from build123d import *

# Parameters (mm, degrees)
BOSS_EXTRUDE1_DEPTH = 6
SKETCH2_R           = 2
CUT_EXTRUDE1_DEPTH  = 121.370262108
SKETCH3_R           = 2
CUT_EXTRUDE2_DEPTH  = 121.370262108
CUT_EXTRUDE3_DEPTH  = 4
SKETCH6_W           = 48
SKETCH6_H           = 40
CUT_EXTRUDE4_DEPTH  = 109.231233939
FILLET1_R           = 5
CHAMFER1_SIZE       = 1


with BuildPart() as part:
    # Sketch1 → Boss-Extrude1 (new, symmetric)
    with BuildSketch(Plane(origin=(0, 0, 0), x_dir=(1, 0, 0), z_dir=(0, 1, 0))):
        Polygon((20, 103), (31, 103), (31, 0), (-31, 0), (-31, 103), (-20, 103), (-20, 10), (20, 10), align=None)
    extrude(amount=BOSS_EXTRUDE1_DEPTH, both=True)

    # Sketch2 → Cut-Extrude1 (cut, through all)
    with BuildSketch(Plane(origin=(31, 0, 0), x_dir=(0, 0, -1), z_dir=(1, 0, 0))):
        with Locations((97, 0)):
            Circle(SKETCH2_R)
        with BuildLine():
            Line((97, 6), (104, 6))
            Line((104, 6), (104, -6))
            Line((104, -6), (97, -6))
            ThreePointArc((97, -6), (103, 0), (97, 6))
        make_face()
    extrude(amount=-CUT_EXTRUDE1_DEPTH, mode=Mode.SUBTRACT)

    # Sketch3 → Cut-Extrude2 (cut, through all)
    with BuildSketch(Plane(origin=(31, 0, 0), x_dir=(0, 0, -1), z_dir=(1, 0, 0))):
        with Locations((18, 0)):
            Circle(SKETCH3_R)
    extrude(amount=-CUT_EXTRUDE2_DEPTH, mode=Mode.SUBTRACT)

    # Sketch4 → Cut-Extrude3 (cut)
    with BuildSketch(Plane(origin=(31, 0, 0), x_dir=(0, 0, -1), z_dir=(1, 0, 0))):
        Polygon((22.041451884, 0), (20.020725942, 3.5), (15.979274058, 3.5), (13.958548116, 0), (15.979274058, -3.5), (20.020725942, -3.5), align=None)
    cut_extrude3 = extrude(amount=-CUT_EXTRUDE3_DEPTH, mode=Mode.SUBTRACT)

    # Mirror1: Cut-Extrude3 across plane
    add(cut_extrude3.mirror(Plane(origin=(0, 0, 0), x_dir=(0, 0, 1), z_dir=(1, 0, 0))), mode=Mode.SUBTRACT)

    # Sketch6 → Cut-Extrude4 (cut, through all)
    with BuildSketch(Plane(origin=(0, 6, 0), x_dir=(1, 0, 0), z_dir=(0, 1, 0))):
        with Locations((0, 30)):
            Rectangle(SKETCH6_W, SKETCH6_H)
    extrude(amount=-CUT_EXTRUDE4_DEPTH, mode=Mode.SUBTRACT)

    # Fillet1
    fillet1_edges = [part.edges().sort_by_distance(p)[0] for p in [
        (31, 0, 0),
        (-31, 0, 0),
    ]]
    fillet(fillet1_edges, radius=FILLET1_R)

    # Chamfer1
    chamfer1_edges = [part.edges().sort_by_distance(p)[0] for p in [
        (-20, -6, -73.5),
        (-20, 6, -73.5),
        (0, -6, 0),
        (0, 6, 0),
        (31, -6, -51),
        (29.535533906, -6, -1.464466094),
        (-29.535533906, -6, -1.464466094),
        (31, 6, -51),
        (29.535533906, 6, -1.464466094),
        (-29.535533906, 6, -1.464466094),
        (0, 6, -10),
        (-31, -6, -51),
        (20, -6, -73.5),
        (-31, 6, -51),
        (20, 6, -73.5),
        (20, 0, -103),
        (-20, 0, -103),
        (-31, 0, -103),
        (31, 0, -103),
        (0, -6, -10),
    ]]
    chamfer(chamfer1_edges, length=CHAMFER1_SIZE)


solid = part.part
Model file for the job. Use its own axes, mm. A direction names the side the tool comes from. Give positions to 0.01 mm unless a question says otherwise; leave off trailing zeros. Order: outer loops, then holes, each group sorted by start corner. A loop starts at its lowest first (then second) coordinate and runs counter-clockwise, first axis right, second up. Notation, with made-up numbers: (55.25, 53.25) - (103.25, 53.25) arc R26 cw to (103.25, 78.25) - close; hole circle Ø5 at (-15, 48). An arc over 180 degrees is marked (long way). Return JSON: item names as keys, results as strings.
1) Pull direction X, two halves, no side cores. Call faces 1 (the flat face through (-22, 6, -53)), 2 (the conical face through (-29.063, 5.715, -2.004)), 3 (the conical face through (20.2, -0.1, -102.2)), 4 (the cylindrical face through (30, 0, -2)): pulls with the +X half, pulls with the -X half, needs draft (parallel to the pull), parting line crosses it, or undercut.
Geometry says:
{"face 1": "needs draft", "face 2": "pulls with the -X half", "face 3": "undercut", "face 4": "pulls with the +X half"}
2) Flat gauge pins, fed straight in: P1, Ø3.5, axis at y = -1, z = -19.5, coming from the +X side; P2, Ø3.5, axis at y = 0, z = -18, coming from the +X side; P3, Ø1, axis at x = 20, y = -2, coming from the -Z side; P4, Ø4.5, axis at y = 0, z = -18, coming from the +X side. Where does each tip first touch, or does it go through?
Geometry says:
{"P1": "x = 31", "P2": "through", "P3": "z = -102.16", "P4": "x = 27"}
3) 3-axis set-ups, long thin cutter, end or side, ignore diameter. For faces 5 (the flat face through (-20, 0, -76)), 6 (the conical face through (-20.2, 0.1, -102.2)), 7 (the flat face through (-29.028, -1.726, -14.955)): which of +Z, -Z, +X, -X, +Y, -Y reach the whole face in a straight line?
Geometry says:
{"face 5": "-Z, +Y, -Y", "face 6": "-Z", "face 7": "-X"}
4) Cut at A-A, the plane z = -34. Give the cut face in (x, y).
Geometry says:
{"outline": "(-31, -5) - (-30, -6) - (-24, -6) - (-24, 6) - (-30, 6) - (-31, 5) - close; (24, -6) - (30, -6) - (31, -5) - (31, 5) - (30, 6) - (24, 6) - close"}
5) Cut at C-C, the plane z = -77.5. Give the cut face in (x, y), plus the area to 3 significant figures.
Geometry says:
{"outline": "(-31, -5) - (-30, -6) - (-21, -6) - (-20, -5) - (-20, 5) - (-21, 6) - (-30, 6) - (-31, 5) - close; (20, -5) - (21, -6) - (30, -6) - (31, -5) - (31, 5) - (30, 6) - (21, 6) - (20, 5) - close", "area": "260 mm²"}
6) Cut at B-B, the plane x = 4. Give the cut face in (y, z), plus the area to 3 significant figures.
Geometry says:
{"outline": "(-6, -9) - (-5, -10) - (5, -10) - (6, -9) - (6, -1) - (5, 0) - (-5, 0) - (-6, -1) - close", "area": "118 mm²"}
7) Probe line 1 (X direction, y = 3, z = -53); line 2 (Y direction, x = 26, z = -97); line 3 (X direction, y = -2.5, z = -26.5). List the from-to ranges inside material, lowest first. Write a range as from..to.
Geometry says:
{"line 1": "-31..-20, 20..31", "line 2": "-6..-2, 2..6", "line 3": "-31..-24, 24..31"}
